```python
from build123d import *

# Parameters (mm, degrees)
SKETCH1_W           = 124
SKETCH1_H           = 84
BOSS_EXTRUDE1_DEPTH = 9.5
SKETCH2_W           = 118
SKETCH2_H           = 78
CUT_EXTRUDE1_DEPTH  = 8
FILLET1_R           = 2
FILLET2_R           = 5
SKETCH3_R           = 6
CUT_EXTRUDE2_DEPTH  = 2
SKETCH4_W           = 30
SKETCH4_H           = 3.5
CUT_EXTRUDE3_DEPTH  = 4
SKETCH5_W           = 10
SKETCH5_H           = 10
BOSS_EXTRUDE2_DEPTH = 8
FILLET3_R           = 3
SKETCH6_R           = 1.6
CUT_EXTRUDE4_DEPTH  = 9.5
SKETCH7_R           = 3
CUT_EXTRUDE5_DEPTH  = 2.5
SKETCH8_W           = 10
SKETCH8_H           = 10
BOSS_EXTRUDE3_DEPTH = 8
FILLET4_R           = 3
SKETCH9_R           = 1.6
CUT_EXTRUDE6_DEPTH  = 9.5
SKETCH10_R          = 3
CUT_EXTRUDE7_DEPTH  = 2


with BuildPart() as part:
    # Sketch1 → Boss-Extrude1 (new body)
    with BuildSketch(Plane(origin=(0, 0, 0), x_dir=(1, 0, 0), z_dir=(0, 1, 0))):
        with Locations((-420.885550013, -74.097210731)):
            Rectangle(SKETCH1_W, SKETCH1_H)
    extrude(amount=BOSS_EXTRUDE1_DEPTH)

    # Sketch2 → Cut-Extrude1 (cut)
    with BuildSketch(Plane.XZ):
        with Locations((-420.885550013, 74.097210731)):
            Rectangle(SKETCH2_W, SKETCH2_H)
    extrude(amount=-CUT_EXTRUDE1_DEPTH, mode=Mode.SUBTRACT)

    # Fillet1
    fillet1_edges = [part.edges().sort_by_distance(p)[0] for p in [
        (-479.885550013, 4, 35.097210731),
        (-479.885550013, 4, 113.097210731),
        (-361.885550013, 4, 113.097210731),
        (-361.885550013, 4, 35.097210731),
    ]]
    fillet(fillet1_edges, radius=FILLET1_R)

    # Fillet2
    fillet2_edges = [part.edges().sort_by_distance(p)[0] for p in [
        (-482.885550013, 4.75, 32.097210731),
        (-358.885550013, 4.75, 32.097210731),
        (-358.885550013, 4.75, 116.097210731),
        (-482.885550013, 4.75, 116.097210731),
    ]]
    fillet(fillet2_edges, radius=FILLET2_R)

    # Sketch3 → Cut-Extrude2 (cut)
    with BuildSketch(Plane(origin=(0, 9.5, 0), x_dir=(1, 0, 0), z_dir=(0, 1, 0))):
        with Locations(Location((-465.885550013, -57.447210731, 0), (0, 0, 270))):
            Circle(SKETCH3_R)
        with Locations(Location((-445.885550013, -57.447210731, 0), (0, 0, 270))):
            Circle(SKETCH3_R)
        with Locations(Location((-425.885550013, -57.447210731, 0), (0, 0, 270))):
            Circle(SKETCH3_R)
        with Locations(Location((-405.885550013, -57.447210731, 0), (0, 0, 270))):
            Circle(SKETCH3_R)
        with Locations(Location((-385.885550013, -57.447210731, 0), (0, 0, 270))):
            Circle(SKETCH3_R)
        with Locations(Location((-465.885550013, -76.447210731, 0), (0, 0, 270))):
            Circle(SKETCH3_R)
        with Locations(Location((-445.885550013, -76.447210731, 0), (0, 0, 270))):
            Circle(SKETCH3_R)
        with Locations(Location((-425.885550013, -76.447210731, 0), (0, 0, 270))):
            Circle(SKETCH3_R)
        with Locations(Location((-405.885550013, -76.447210731, 0), (0, 0, 270))):
            Circle(SKETCH3_R)
        with Locations(Location((-385.885550013, -76.447210731, 0), (0, 0, 270))):
            Circle(SKETCH3_R)
        with Locations(Location((-465.885550013, -95.447210731, 0), (0, 0, 270))):
            Circle(SKETCH3_R)
        with Locations(Location((-445.885550013, -95.447210731, 0), (0, 0, 270))):
            Circle(SKETCH3_R)
        with Locations(Location((-405.885550013, -95.447210731, 0), (0, 0, 270))):
            Circle(SKETCH3_R)
        with Locations(Location((-385.885550013, -95.447210731, 0), (0, 0, 270))):
            Circle(SKETCH3_R)
    extrude(amount=-CUT_EXTRUDE2_DEPTH, mode=Mode.SUBTRACT)

    # Sketch4 → Cut-Extrude3 (cut)
    with BuildSketch(Plane(origin=(0, 0, 32.097210731), x_dir=(-1, 0, 0), z_dir=(0, 0, -1))):
        with Locations((390.885550013, 1.75)):
            Rectangle(SKETCH4_W, SKETCH4_H)
        with Locations((450.885550013, 1.75)):
            Rectangle(SKETCH4_W, SKETCH4_H)
    extrude(amount=-CUT_EXTRUDE3_DEPTH, mode=Mode.SUBTRACT)

    # Sketch5 → Boss-Extrude2 (add)
    with BuildSketch(Plane.XZ.offset(-8)):
        with Locations((-474.885550013, 108.097210731)):
            Rectangle(SKETCH5_W, SKETCH5_H)
        with Locations((-366.885550013, 108.097210731)):
            Rectangle(SKETCH5_W, SKETCH5_H)
        with Locations((-366.885550013, 40.097210731)):
            Rectangle(SKETCH5_W, SKETCH5_H)
        with Locations((-474.885550013, 40.097210731)):
            Rectangle(SKETCH5_W, SKETCH5_H)
    extrude(amount=BOSS_EXTRUDE2_DEPTH)

    # Fillet3
    fillet3_edges = [part.edges().sort_by_distance(p)[0] for p in [
        (-469.885550013, 4, 103.097210731),
        (-371.885550013, 4, 103.097210731),
        (-371.885550013, 4, 45.097210731),
        (-469.885550013, 4, 45.097210731),
    ]]
    fillet(fillet3_edges, radius=FILLET3_R)

    # Sketch6 → Cut-Extrude4 (cut)
    with BuildSketch(Plane.XZ):
        with Locations(Location((-475.885550013, 109.097210731, 0), (0, 0, 270))):
            Circle(SKETCH6_R)
        with Locations(Location((-365.885550013, 109.097210731, 0), (0, 0, 270))):
            Circle(SKETCH6_R)
        with Locations(Location((-365.885550013, 39.097210731, 0), (0, 0, 270))):
            Circle(SKETCH6_R)
        with Locations(Location((-475.885550013, 39.097210731, 0), (0, 0, 270))):
            Circle(SKETCH6_R)
    extrude(amount=-CUT_EXTRUDE4_DEPTH, mode=Mode.SUBTRACT)

    # Sketch7 → Cut-Extrude5 (cut)
    with BuildSketch(Plane(origin=(0, 9.5, 0), x_dir=(1, 0, 0), z_dir=(0, 1, 0))):
        with Locations(Location((-365.885550013, -39.097210731, 0), (0, 0, 270))):
            Circle(SKETCH7_R)
        with Locations(Location((-365.885550013, -109.097210731, 0), (0, 0, 270))):
            Circle(SKETCH7_R)
        with Locations(Location((-475.885550013, -109.097210731, 0), (0, 0, 270))):
            Circle(SKETCH7_R)
        with Locations(Location((-475.885550013, -39.097210731, 0), (0, 0, 270))):
            Circle(SKETCH7_R)
    extrude(amount=-CUT_EXTRUDE5_DEPTH, mode=Mode.SUBTRACT)

    # Sketch8 → Boss-Extrude3 (add)
    with BuildSketch(Plane.XZ.offset(-8)):
        with Locations((-420.885550013, 40.097210731)):
            Rectangle(SKETCH8_W, SKETCH8_H)
        with Locations((-420.885550013, 108.097210731)):
            Rectangle(SKETCH8_W, SKETCH8_H)
    extrude(amount=BOSS_EXTRUDE3_DEPTH)

    # Fillet4
    fillet4_edges = [part.edges().sort_by_distance(p)[0] for p in [
        (-425.885550013, 4, 45.097210731),
        (-415.885550013, 4, 45.097210731),
        (-425.885550013, 4, 103.097210731),
        (-415.885550013, 4, 103.097210731),
    ]]
    fillet(fillet4_edges, radius=FILLET4_R)

    # Sketch9 → Cut-Extrude6 (cut)
    with BuildSketch(Plane.XZ):
        with Locations(Location((-420.885550013, 39.097210731, 0), (0, 0, 270))):
            Circle(SKETCH9_R)
        with Locations(Location((-420.885550013, 109.097210731, 0), (0, 0, 270))):
            Circle(SKETCH9_R)
    extrude(amount=-CUT_EXTRUDE6_DEPTH, mode=Mode.SUBTRACT)

    # Sketch10 → Cut-Extrude7 (cut)
    with BuildSketch(Plane(origin=(0, 9.5, 0), x_dir=(1, 0, 0), z_dir=(0, 1, 0))):
        with Locations(Location((-420.885550013, -109.097210731, 0), (0, 0, 270))):
            Circle(SKETCH10_R)
        with Locations(Location((-420.885550013, -39.097210731, 0), (0, 0, 270))):
            Circle(SKETCH10_R)
    extrude(amount=-CUT_EXTRUDE7_DEPTH, mode=Mode.SUBTRACT)


solid = part.part
```
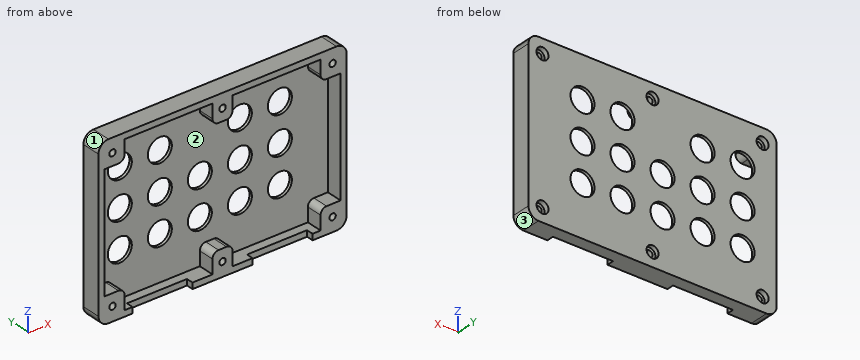
Input: part model. Units: mm. Frame: model coordinates. Face numbers are marked on the shaded views. Round coordinates to 2 decimals unless told otherwise and drop trailing zeros. Write each loop counter-clockwise with the first axis right and the second up, starting at its lowest first coordinate (ties: lowest second). Pieces come first, ordered by that corner, then holes. Notation, with made-up numbers: M 44.5,76 L 77.5,76 A13 ccw 77.5,92 Z; hole C 26,83 d5. An arc over 180 degrees is marked long. Write each question's results on one line, items separated by ' | '.
Q1. Section query A-A (z = 98). Return loops of the section in (x, y), and give its area (3 significant figures).
Results:
outline: M -482.89,0 L -479.89,0 L -479.89,8 L -471.32,8 L -471.32,9.5 L -482.89,9.5 Z; M -460.46,8 L -451.32,8 L -451.32,9.5 L -460.46,9.5 Z; M -440.46,8 L -411.32,8 L -411.32,9.5 L -440.46,9.5 Z; M -400.46,8 L -391.32,8 L -391.32,9.5 L -400.46,9.5 Z; M -380.46,8 L -361.89,8 L -361.89,0 L -358.89,0 L -358.89,9.5 L -380.46,9.5 Z | area: 169 mm^2
Q2. Section query B-B (x = -378.5). Return loops of the section in (y, z).
Results:
outline: M 0,113.1 L 8,113.1 L 8,35.1 L 3.5,35.1 L 3.5,32.1 L 9.5,32.1 L 9.5,116.1 L 0,116.1 Z
Q3. Pin query (flat end, axial travel): P1, Ø11, axis at x = -445.89, z = 95.45, coming from the -Y side; P2, Ø19, axis at x = -405.89, z = 95.45, coming from the -Y side; P3, Ø3.5, axis at y = 1.5, z = 34, coming from the -X side; P4, Ø1, axis at x = -455, y = 1, coming from the -Z side. Return the tip coordinate at first contact, or that it passes through.
Results:
P1: passes through | P2: stops at y = 8 | P3: stops at x = -482.7 | P4: stops at z = 113.1
Q4. Line query: line 1 along Z through (x, y) = (-469.5, 2.25); line 2 along Z through (x, y) = (-368.5, 6.5); line 3 along X through (y, z) = (6.25, 72). Output: solid intervals per line, ascending.
Results:
line 1: z = 32.1 to 35.1, 113.1 to 116.1 | line 2: z = 32.1 to 45.1, 103.1 to 116.1 | line 3: x = -482.89 to -479.89, -361.89 to -358.89
Q5. Section query D-D (x = -408.5). Return loops of the section in (y, z).
Results:
outline: M 0,32.1 L 9.5,32.1 L 9.5,52.05 L 8,52.05 L 8,35.1 L 0,35.1 Z; M 0,113.1 L 8,113.1 L 8,100.85 L 9.5,100.85 L 9.5,116.1 L 0,116.1 Z; M 8,62.85 L 9.5,62.85 L 9.5,71.05 L 8,71.05 Z; M 8,81.85 L 9.5,81.85 L 9.5,90.05 L 8,90.05 Z
Q6. Section query C-C (z = 87). Return loops of the section in (x, y).
Results:
outline: M -482.89,0 L -479.89,0 L -479.89,8 L -361.89,8 L -361.89,0 L -358.89,0 L -358.89,9.5 L -482.89,9.5 Z
Q7. Draft query along X for the marked faces 1, 2 and 3. Return one class per face: released by +X, released by -X, zero draft, split by the parting line, or undercut.
Results:
face 1: released by -X | face 2: undercut | face 3: released by +X
